from build123d import *

# Parameters (mm, degrees)
SKETCH1_R           = 14.3002
BOSS_EXTRUDE1_DEPTH = 6.35
FILLET1_R           = 10.16
FILLET2_R           = 12.7


with BuildPart() as part:
    # Sketch1 → Boss-Extrude1 (new body)
    with BuildSketch(Plane.XY):
        with BuildLine():
            Line((-78.624201442, -19.05), (0, -19.05))
            ThreePointArc((0, -19.05), (15.29709191, 11.353478722), (-18.233617587, 5.517036315))
            ThreePointArc((-18.233617587, 5.517036315), (-97.907934324, 238.196201056), (143.154480855, 286.945585057))
            ThreePointArc((143.154480855, 286.945585057), (178.751803486, 291.757091583), (173.940297689, 327.354414313))
            ThreePointArc((173.940297689, 327.354414313), (-27.542038168, 358.917389173), (-164.282230707, 207.611497719))
            Line((-164.282230707, 207.611497719), (-215.082230707, 207.611497719))
            Line((-215.082230707, 207.611497719), (-215.082230707, 106.011497719))
            Line((-215.082230707, 106.011497719), (-164.282230707, 106.011497719))
            ThreePointArc((-164.282230707, 106.011497719), (-132.874579252, 35.657945846), (-78.624201442, -19.05))
        make_face()
        Circle(SKETCH1_R, mode=Mode.SUBTRACT)
        with Locations((158.547388858, 307.15)):
            Circle(SKETCH1_R, mode=Mode.SUBTRACT)
    extrude(amount=BOSS_EXTRUDE1_DEPTH)

    # Fillet1
    fillet1_edges = [part.edges().sort_by_distance(p)[0] for p in [
        (-78.624201442, -19.05, 3.175),
        (-164.282230707, 106.011497719, 3.175),
        (-164.282230707, 207.611497719, 3.175),
    ]]
    fillet(fillet1_edges, radius=FILLET1_R)

    # Fillet2
    fillet2_edges = [part.edges().sort_by_distance(p)[0] for p in [
        (-18.233617587, 5.517036315, 3.175),
    ]]
    fillet(fillet2_edges, radius=FILLET2_R)


solid = part.part
Design review of the part built by this model. Coordinates are the model's own, in mm. Round coordinates to 2 decimals unless told otherwise and drop trailing zeros. Write each loop counter-clockwise with the first axis right and the second up, starting at its lowest first coordinate (ties: lowest second). Pieces come first, ordered by that corner, then holes. Notation, with made-up numbers: (62, -38) - (79, -38) arc R25 ccw to (79, -18) - close; hole circle Ø4 at (73.5, 43.25). An arc over 180 degrees is marked (long way). Use a Markdown table: item, result. Add a question column.
1. We need section C-C (y = 0). State the section outline as (x, z) points, then the cut area to 3 significant figures.
2. We need section A-A (y = 307.15). State the section outline as (x, z) points.
3. We need section D-D (z = 2.75). Count the separate pieces of the cut face and the enclosed holes in it, then the cut area to 3 significant figures.
4. Mouldability with a two-part tool opening along Y and no side actions: class faces 1 (the face through (-105, 235, 0)), 2 (the face through (156.69, 321.33, 3.13)), 3 (the face through (-21.146, 361.069, 3.131)) as +Y half, -Y half, draft (parallel to the pull), parting line (faces both ways), or undercut.
5. We need section B-B (x = -57). State the section outline as (y, z) points.
6. Clearance check with flat-ended pins moving along their axes: pin 1 (3 mm diameter, centred on y = 218.5, z = 4.5, fed in from +X); pin 2 (3 mm diameter, centred on x = -195, z = 4, fed in from +Y); pin 3 (1 mm diameter, centred on x = 69, z = 4.5, fed in from +Y). State where each tip first meets the part, or that it passes through.
7. Wall thickness on probe 1 along Y at (x, z) = (7.5, 4); probe 2 along Y at (x, z) = (0, 2.75); probe 3 along X at (y, z) = (7.5, 2): over which ranges is each line inside the solid? List them lowest first.
Output:
| question | item | result |
|---|---|---|
| 1 | outline | (-102.2, 0) - (-14.3, 0) - (-14.3, 6.35) - (-102.2, 6.35) - close; (14.3, 0) - (19.05, 0) - (19.05, 6.35) - (14.3, 6.35) - close |
| 1 | area | 588 mm2 |
| 2 | outline | (-108.85, 0) - (-20.51, 0) - (-20.51, 6.35) - (-108.85, 6.35) - close; (108.53, 0) - (144.25, 0) - (144.25, 6.35) - (108.53, 6.35) - close; (172.85, 0) - (183.95, 0) - (183.95, 6.35) - (172.85, 6.35) - close |
| 3 | separate pieces | 1 |
| 3 | enclosed holes | 2 |
| 3 | area | 37,900 mm2 |
| 4 | face 1 | draft |
| 4 | face 2 | undercut |
| 4 | face 3 | +Y half |
| 5 | outline | (-19.05, 0) - (28.12, 0) - (28.12, 6.35) - (-19.05, 6.35) - close; (285.5, 0) - (345.92, 0) - (345.92, 6.35) - (285.5, 6.35) - close |
| 6 | pin 1 | stops at x = -106.89 |
| 6 | pin 2 | stops at y = 207.61 |
| 6 | pin 3 | stops at y = 369.81 |
| 7 | probe 1 | y = -17.51 to -12.18, 12.18 to 17.51, 316.28 to 368.08 |
| 7 | probe 2 | y = -19.05 to -14.3, 14.3 to 19.05, 314.38 to 366.64 |
| 7 | probe 3 | x = -109.85 to -12.18, 12.18 to 17.51 |
